Part model, mm, in its own coordinate system. A direction names the side the tool comes from. Coordinates: 2 decimals unless noted, no trailing zeros. Loops run counter-clockwise (first coordinate to the right, second up) from the corner with the lowest first, then second, coordinate; pieces in that order, holes last. Notation, with made-up numbers: (-33, -25.75) - (-8, -25.75) arc R22 ccw to (-8, -7.75) - close; hole circle Ø6 at (-1, 41). An arc over 180 degrees is marked (long way). One line per question, with ' | ' between items. Start each with the question number.
from build123d import *

# Parameters (mm, degrees)
F0_R     = 33.8455
F0_R_2   = 29.083
F1_DEPTH = 31.75
F0_R_3   = 25.273
F2_DEPTH = 7.9375
F3_R     = 30.1625
F3_R_2   = 25.4
F4_DEPTH = 6.35
F5_SIZE  = 2.54


with BuildPart() as f1:
    # F0 (on Top) → F1 (new body)
    with BuildSketch(Plane.XY):
        Circle(F0_R)
        Circle(F0_R_2, mode=Mode.SUBTRACT)
    extrude(amount=F1_DEPTH)

    # F0 (on Top) → F2 (join)
    with BuildSketch(Plane.XY):
        Circle(F0_R)
        Circle(F0_R_2, mode=Mode.SUBTRACT)
        Circle(F0_R_2)
        Circle(F0_R_3, mode=Mode.SUBTRACT)
    extrude(amount=-F2_DEPTH)

    # F3 (on face) → F4 (join)
    with BuildSketch(Plane(origin=(0, 0, -7.9375), x_dir=(1, 0, 0), z_dir=(0, 0, -1))):
        Circle(F3_R)
        Circle(F3_R_2, mode=Mode.SUBTRACT)
    extrude(amount=F4_DEPTH)

    # F5
    f5_edges = [f1.edges().sort_by_distance(p)[0] for p in [
        (-33.8455, 0, 31.75),
        (-33.8455, 0, -7.9375),
        (-30.1625, 0, -14.2875),
    ]]
    chamfer(f5_edges, length=F5_SIZE)


solid = f1.part
1) Tool access for faces 1 (the flat face through (-16, 26, -7.938)), 2 (the flat face through (9, -28, 31.75)), 3 (the flat face through (-9, 24, 0)): list every direction of +Z, -Z, +X, -X, +Y, -Y with a clear straight run to the whole face (end or side of a thin tool).
2) Mould opens along X. For faces 4 (the cylindrical face through (-5.506, 24.796, -11.068)), 5 (the cylindrical face through (-30.133, -1.326, -9.816)), 6 (the flat face through (8.1, 24.4, -14.288)) say: +X half, -X half, draft (parallel to the pull), parting line (faces both ways), or undercut.
3) Wall check: line 1 along Y through (x, z) = (0, -10.75); line 2 along Y through (x, z) = (0, -3). Give the ranges that are in metal, low to high. Write a range as [from, to].
4) Band-saw the part on A-A on y = 0. List the corners of the cut face in (x, z), then the cut area to 3 significant figures.
5) Pin check, flat tips, straight feed: pin 1 Ø8 at (x, y) = (0.5, 22) entering from -Z; pin 2 Ø12 at (y, z) = (-19.5, -5.5) entering from +X; pin 3 Ø5 at (x, z) = (9.5, 1) entering from +Y; pin 4 Ø10 at (y, z) = (17, 11.5) entering from +X. Stop position of each tip, or through.
6) Band-saw the part on C-C on z = 19. List the corners of the cut face in (x, y), then the cut area to 3 significant figures.
Values found:
1) face 1: -Z | face 2: +Z, +X, -X, +Y, -Y | face 3: +Z
2) face 4: undercut | face 5: parting line | face 6: draft
3) line 1: [-30.16, -25.4], [25.4, 30.16] | line 2: [-33.85, -25.27], [25.27, 33.85]
4) outline: (-33.85, -5.4) - (-31.31, -7.94) - (-30.16, -7.94) - (-30.16, -11.75) - (-27.62, -14.29) - (-25.4, -14.29) - (-25.4, -7.94) - (-25.27, -7.94) - (-25.27, 0) - (-29.08, 0) - (-29.08, 31.75) - (-31.31, 31.75) - (-33.85, 29.21) - close; (25.27, -7.94) - (25.4, -7.94) - (25.4, -14.29) - (27.62, -14.29) - (30.16, -11.75) - (30.16, -7.94) - (31.31, -7.94) - (33.85, -5.4) - (33.85, 29.21) - (31.31, 31.75) - (29.08, 31.75) - (29.08, 0) - (25.27, 0) - close | area: 480 mm²
5) pin 1: z = -14.29 | pin 2: x = 31.04 | pin 3: y = 33.11 | pin 4: x = 31.65
6) outline: circle Ø67.69 at (0, 0); hole circle Ø58.17 at (0, 0) | area: 942 mm²
